Verification items for the finished model (mm, model axes). A direction names the side the tool comes from. Round coordinates to 2 decimals unless told otherwise and drop trailing zeros. Loops run counter-clockwise (first coordinate to the right, second up) from the corner with the lowest first, then second, coordinate; pieces in that order, holes last. Notation, with made-up numbers: (26, 80.25) - (62, 80.25) arc R29 cw to (62, 114.25) - close; hole circle Ø1 at (15, 24). An arc over 180 degrees is marked (long way). Use CSV: the item, a comma, the result in double quotes.
```python
from build123d import *

# Parameters (mm, degrees)
BOSS_EXTRUDE1_DEPTH     = 4.7625
F_1_4_CLEARANCE_HOLE4_D = 6.5278
M4_CLEARANCE_HOLE1_D    = 4.3
F_1_4_20_TAPPED_HOLE1_D = 5.1054


with BuildPart() as part:
    # Sketch2 → Boss-Extrude1 (new body)
    with BuildSketch(Plane(origin=(0, 0, 0), x_dir=(1, 0, 0), z_dir=(0, 1, 0))):
        with BuildLine():
            Line((144.946020413, 76.679156198), (7.085990937, 128.90997287))
            ThreePointArc((7.085990937, 128.90997287), (0.000172842, 130.207283228), (-7.085650583, 128.910001974))
            Line((-7.085650583, 128.910001974), (-144.945894589, 76.679751543))
            ThreePointArc((-144.945894589, 76.679751543), (-150.520615414, 71.435599421), (-150.754362786, 63.785500995))
            Line((-150.754362786, 63.785500995), (-129.497015734, 7.677344758))
            ThreePointArc((-129.497015734, 7.677344758), (-124.252863612, 2.102623932), (-116.602765186, 1.86887656))
            Line((-116.602765186, 1.86887656), (-3.542913137, 44.703157239))
            ThreePointArc((-3.542913137, 44.703157239), (-1.425e-06, 45.351797866), (3.542907623, 44.703142687))
            Line((3.542907623, 44.703142687), (116.602583736, 1.868397631))
            ThreePointArc((116.602583736, 1.868397631), (124.252683122, 2.102113581), (129.496858142, 7.676812867))
            Line((129.496858142, 7.676812867), (150.75443565, 63.784881792))
            ThreePointArc((150.75443565, 63.784881792), (150.520719699, 71.434981178), (144.946020413, 76.679156198))
        make_face()
    extrude(amount=-BOSS_EXTRUDE1_DEPTH)

    # 1/4 Clearance Hole4 (through all)
    with Locations(Plane(origin=(0, 0, 0), x_dir=(1, 0, 0), z_dir=(0, 1, 0))):
        with Locations((84.499786461, 52.795924918), (-84.499851108, 52.795924918)):
            Hole(F_1_4_CLEARANCE_HOLE4_D / 2)

    # M4 Clearance Hole1 (through all)
    with Locations(Plane(origin=(0, 0, 0), x_dir=(1, 0, 0), z_dir=(0, 1, 0))):
        with Locations((-49.61075086, 66.014140629), (-119.745946152, 39.442456816), (49.610666218, 66.014000002), (119.745752362, 39.442028122)):
            Hole(M4_CLEARANCE_HOLE1_D / 2)

    # 1/4-20 Tapped Hole1 (through all)
    with Locations(Plane(origin=(0, 0, 0), x_dir=(1, 0, 0), z_dir=(0, 1, 0))):
        with Locations((-2.901e-06, 111.151797866), (-2.901e-06, 60.351797866)):
            Hole(F_1_4_20_TAPPED_HOLE1_D / 2)


solid = part.part
```
1) Cross-section at D-D, the plane z = -98. Record the cut outline in (x, y).
Returned:
outline,"(-88.67, -4.76) - (88.67, -4.76) - (88.67, 0) - (-88.67, 0) - close"
2) Gauge pin test, flat ends, axial feed: pin 1 Ø2 at (x, y) = (111.5, -3.5) entering from -Z; pin 2 Ø4.5 at (x, z) = (0, -111.15) entering from -Y; pin 3 Ø1.5 at (y, z) = (-4, -49.5) entering from -X; pin 4 Ø1.5 at (x, y) = (103, -3.5) entering from -Z. Record the tip position at first contact, or that the pin passes through.
Returned:
pin 1,"stops at z = -89.73"
pin 2,"passes through"
pin 3,"stops at x = -145.63"
pin 4,"stops at z = -92.86"
3) Cross-section at C-C, the plane x = 84. Record the cut outline in (y, z), then the cut area to 3 significant figures.
Returned:
outline,"(-4.76, -99.77) - (0, -99.77) - (0, -56.02) - (-4.76, -56.02) - close; (-4.76, -49.57) - (0, -49.57) - (0, -14.22) - (-4.76, -14.22) - close"
area,"377 mm²"
4) Mould release check, pull along X, two halves, no side actions. Record for faces 3 (the face through (-75.05, -2.35, -103.16)), 4 (the face through (-60.864, -2.348, -22.986)), 5 (the face through (124.152, -2.348, -2.058)), 6 (the face through (-2, 0, -67)): +X half, -X half, draft (parallel to the pull), parting line (faces both ways), or undercut.
Returned:
face 3,"-X half"
face 4,"undercut"
face 5,"undercut"
face 6,"draft"
5) Cross-section at A-A, the plane z = -22.5. Record the cut outline in (x, y).
Returned:
outline,"(-135.11, -4.76) - (-62.15, -4.76) - (-62.15, 0) - (-135.11, 0) - close; (62.15, -4.76) - (135.11, -4.76) - (135.11, 0) - (62.15, 0) - close"
6) Access from +Z, -Z, +X, -X, +Y, -Y to the whole of each face (thin tool, end or side, straight path). Record for faces 1 (the face through (81.387, -2.415, -53.776)), 2 (the face through (59.281, -2.348, -23.586)).
Returned:
face 1,"+Y, -Y"
face 2,"+Z, +Y, -Y"
7) Thickness scan on probe 1 along X at (y, z) = (-1.2, -48.5); probe 2 along Z at (x, y) = (-84, -1.15); probe 3 along Z at (x, y) = (1, -3.4). Record the ranges inside material, lowest first. Write a range as [from, to].
Returned:
probe 1,"x = [-144.96, 144.96]"
probe 2,"z = [-99.77, -56.02], [-49.57, -14.22]"
probe 3,"z = [-130.18, -113.5], [-108.8, -62.7], [-58, -45.3]"
8) Cross-section at B-B, the plane y = -3.4. Count the separate pieces of the cut face and the enclosed holes in it, then the cut area to 3 significant figures.
Returned:
separate pieces,"1"
enclosed holes,"8"
area,"23,700 mm²"
